Geometry check sheet. Reference: the model listing, model coordinates, mm. A direction names the side the tool comes from. Round coordinates to 2 decimals unless told otherwise and drop trailing zeros. Write each loop counter-clockwise with the first axis right and the second up, starting at its lowest first coordinate (ties: lowest second). Pieces come first, ordered by that corner, then holes. Notation, with made-up numbers: M 12.25,16.25 L 42.25,16.25 A33 ccw 42.25,49.25 Z; hole C -24.75,81 d3. An arc over 180 degrees is marked long. Put each result on its own line as item: value. Start each with the question number.
(1) Section check D-D on y = -35.5. Record the cut outline in (x, z), then the cut area to 3 significant figures.
(2) Tool access check on faces 1 (the flat face through (1.407, -28.892, 31.955)), 2 (the flat face through (1.45, -37.32, -10.69)), 3 (the flat face through (-1, 0, 0)). Record the directions out of +Z, -Z, +X, -X, +Y, -Y that give a thin tool (end or side, any length) a straight path to the whole face; none if there is none.
(3) Material ranges on probe 1 along X at (y, z) = (-34.5, -12); probe 2 along Z at (x, y) = (73, 6); probe 3 along Y at (x, z) = (-36.5, -31.5), recorded low to high.
(4) Gauge pin test, flat ends, axial feed: pin 1 (4 mm diameter, centred on x = 6.5, y = -33, fed in from -Z); pin 2 (12 mm diameter, centred on x = 19.5, z = -4.5, fed in from -Y); pin 3 (1.5 mm diameter, centred on x = 9.5, y = -29, fed in from +Z). Record the tip position at first contact, or that the pin passes through.
(5) Section check A-A on y = -17. Record the cut outline in (x, z), then the cut area to 3 significant figures.
(6) Mould release check, pull along Y, two halves, no side actions. Record for faces 4 (the flat face through (-100.5, -20, 0)), 5 (the flat face through (1.45, -45.08, 20.21)), 6 (the flat face through (-1, -8, -38.5)), 7 (the flat face through (100.5, -21, 0)): pulls with the +Y half, pulls with the -Y half, needs draft (parallel to the pull), parting line crosses it, or undercut.
(7) Section check B-B on z = -26. Record the cut outline in (x, y).
(8) Section check C-C on x = 83. Record the cut outline in (y, z), then the cut area to 3 significant figures.
from build123d import *

# Parameters (mm, degrees)
F0_W          = 201
F0_H          = 71
F1_DEPTH      = 3
F0_W_2        = 207
F0_H_2        = 77
F2_DEPTH      = 25
F2_DEPTH_BACK = 10
F4_DEPTH      = 3
F5_DEPTH      = 207
F7_DEPTH      = 3
F8_W          = 186.1692070961
F8_H          = 16.862899065
F9_DEPTH      = 2.2177692789


with BuildPart() as f1:
    # F0 (on Front) → F1 (new body)
    with BuildSketch(Plane.XZ):
        Rectangle(F0_W, F0_H)
    extrude(amount=F1_DEPTH)

    # F0 (on Front) → F2 (join, two sides)
    with BuildSketch(Plane.XZ) as f2_sk:
        Rectangle(F0_W_2, F0_H_2)
        Rectangle(F0_W, F0_H, mode=Mode.SUBTRACT)
    extrude(amount=F2_DEPTH)
    extrude(f2_sk.sketch, amount=-F2_DEPTH_BACK)

    # F3 (on face) → F4 (join, through all)
    with BuildSketch(Plane.YZ.offset(103.5)):
        Polygon((-47.4088080227, 15.086744912), (-25, -35.5), (-25, 35.5), align=None)
        Polygon((-49.3025101092, 16.3616811017), (-25, -38.5), (-25, -35.5), (-47.4088080227, 15.086744912), (-25, 35.5), (-25, 38.5), align=None)
    extrude(amount=-F4_DEPTH)

    # F3 (on face) → F5 (join, through all)
    with BuildSketch(Plane.YZ.offset(103.5)):
        Polygon((-49.3025101092, 16.3616811017), (-25, -38.5), (-25, -35.5), (-47.4088080227, 15.086744912), (-25, 35.5), (-25, 38.5), align=None)
    extrude(amount=-F5_DEPTH)

    # F6 (on face) → F7 (join, through all)
    with BuildSketch(Plane(origin=(-103.5, 0, 0), x_dir=(0, -1, 0), z_dir=(-1, 0, 0))):
        Polygon((25, 35.5), (25, -35.5), (47.4088080227, 15.086744912), align=None)
    extrude(amount=-F7_DEPTH)

    # F8 (on face) → F9 (cut, through all)
    with BuildSketch(Plane(origin=(0, -30.504070767, 33.4860786671), x_dir=(1, 0, 0), z_dir=(0, -0.6734240389, 0.7392564263))):
        with Locations((0, -8.4314495325)):
            Rectangle(F8_W, F8_H)
    extrude(amount=-F9_DEPTH, mode=Mode.SUBTRACT)


solid = f1.part
Answers follow:
1. outline: M -103.5,-14.8 L 103.5,-14.8 L 103.5,28.94 L 93.08,28.94 L 93.08,25.94 L 100.5,25.94 L 100.5,-11.8 L -100.5,-11.8 L -100.5,25.94 L -93.08,25.94 L -93.08,28.94 L -103.5,28.94 Z
1. area: 910 mm^2
2. face 1: none
2. face 2: -Z, +X, -X, -Y
2. face 3: +Y
3. probe 1: x = -103.5 to -100.5, 100.5 to 103.5
3. probe 2: z = -38.5 to -35.5, 35.5 to 38.5
3. probe 3: y = -28.1 to -26.77, -3 to 0
4. pin 1: stops at z = -24.96
4. pin 2: stops at y = -42.72
4. pin 3: stops at z = 35.54
5. outline: M -103.5,-38.5 L 103.5,-38.5 L 103.5,38.5 L -103.5,38.5 Z; hole M -100.5,-35.5 L 100.5,-35.5 L 100.5,35.5 L -100.5,35.5 Z
5. area: 1,670 mm^2
6. face 4: undercut
6. face 5: pulls with the -Y half
6. face 6: needs draft
6. face 7: undercut
7. outline: M -103.5,-30.54 L 103.5,-30.54 L 103.5,10 L 100.5,10 L 100.5,0 L -100.5,0 L -100.5,10 L -103.5,10 Z; hole M -100.5,-29.21 L 100.5,-29.21 L 100.5,-3 L -100.5,-3 Z
8. outline: M -49.3,16.36 L -25,-38.5 L 10,-38.5 L 10,-35.5 L 0,-35.5 L 0,35.5 L 10,35.5 L 10,38.5 L -25,38.5 L -30.5,33.49 L -29.01,31.85 L -25,35.5 L -3,35.5 L -3,-35.5 L -25,-35.5 L -47.41,15.09 L -41.48,20.49 L -42.97,22.13 Z
8. area: 526 mm^2
